Model file for the job. Use its own axes, mm. Face numbers are marked on the shaded views. A direction names the side the tool comes from. Round coordinates to 2 decimals unless told otherwise and drop trailing zeros. Loops run counter-clockwise (first coordinate to the right, second up) from the corner with the lowest first, then second, coordinate; pieces in that order, holes last. Notation, with made-up numbers: M 2.25,-29.75 L 54.25,-29.75 A19 ccw 54.25,2.25 Z; hole C -21,-37.75 d10. An arc over 180 degrees is marked long. Use a Markdown table: item, result. Add a question column.
Item 1: Saw through at B-B on x = 18.5. Write the cut outline in (y, z), then the cut area to 3 significant figures.
Item 2: Saw through at D-D on z = 48. Write the cut outline in (x, y) (3 decimals), then the cut area to 3 significant figures.
Item 3: Two-plate mould, pull along Z, no slides. Class the marked faces 1 and 2: +Z half, -Z half, draft (parallel to the pull), parting line (faces both ways), or undercut.
Item 4: Pin check, flat tips, straight feed: P1, Ø8, axis at x = 11.5, z = 59.5, coming from the -Y side; P2, Ø4, axis at y = 38.1, z = 6.35, coming from the +X side; P3, Ø10, axis at x = 17.5, z = 0.5, coming from the -Y side; P4, Ø8.5, axis at y = 38.1, z = 57.15, coming from the +X side (3 decimals). Stop position of each tip, or through.
Item 5: Saw through at C-C on z = 5. Write the cut outline in (x, y) (1 decimal), then the cut area to 3 significant figures.
Item 6: Wall check: L1, parallel to Z at x = 2.2, y = 38.1 (3 decimals); L2, parallel to Y at x = 1.2, z = 57.15 (3 decimals); L3, parallel to X at y = 22.5, z = 49 (3 decimals). Give the ranges that are in metal, low to high. Write a range as from..to.
Item 7: Saw through at A-A on y = 38.1. Write the cut outline in (x, z) (3 decimals).
Item 8: Tool access for the marked faces 3, 4 and 5: list every direction of +Z, -Z, +X, -X, +Y, -Y with a clear straight run to the whole face (end or side of a thin tool).
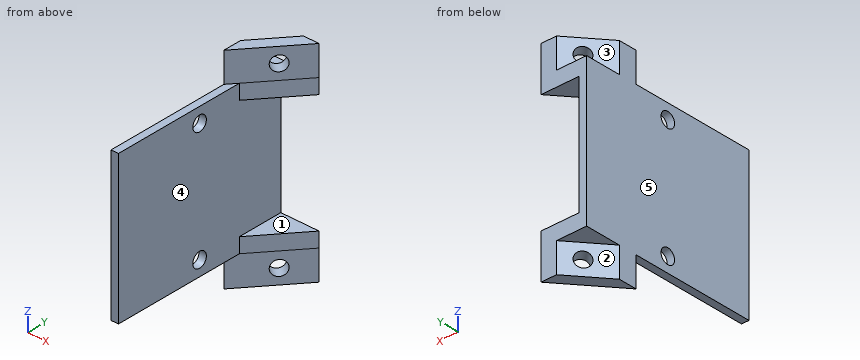
Autodesk Inventor part; units mm, degrees
ref_plane "YZ Plane" through (0, 0, 0) normal (1, 0, 0) x (0, 1, 0)
ref_plane "XZ Plane" through (0, 0, 0) normal (0, 1, 0) x (-1, 0, 0)
ref_plane "XY Plane" through (0, 0, 0) normal (0, 0, 1) x (1, 0, 0)
sketch "Sketch1" plane through (0, 0, 0) normal (1, 0, 0) x (0, 1, 0)
  line L0 (76.2, 63.5) -> (0, 63.5)
  line L1 (0, 63.5) -> (0, 0)
  line L2 (0, 0) -> (76.2, 0)
  line L3 (76.2, 0) -> (76.2, 63.5)
  dimension "d0" = 76.2
  dimension "d1" = 63.5
extrude "Extrusion1" add sketch "Sketch1" along normal blind 3.175
sketch "Sketch2" plane through (3.175, 0, 0) normal (1, 0, 0) x (0, 0, -1)
  line L0 (-63.5, 76.2) -> (-63.5, 0)
  line L1 (0, 0) -> (0, 76.2)
  line L2 (0, 76.2) -> (-63.5, 76.2)
  point P0 (-57.15, 38.1)
  point P1 (-6.35, 38.1)
  dimension "d11" = 6.35
  dimension "d12" = 6.35
  dimension "d13" = 38.1
  dimension "d14" = 38.1
hole "Hole1" at (3.175, 38.1, 57.15) at (3.175, 38.1, 6.35) direction (-1, 0, 0) diameter 6.35 end through all
sketch "Sketch3" plane through (0, 0, 0) normal (0, 0, -1) x (-1, 0, 0)
  line L0 (-19.5018, 76.2) -> (-3.175, 56.7425)
  line L1 (-3.175, 56.7425) -> (-3.175, 76.2)
  line L2 (-3.175, 0) -> (-3.175, 76.2)
  line L3 (-3.175, 76.2) -> (-19.5018, 76.2)
  line L4 (0, 76.2) -> (-3.175, 76.2)
  point P0 (0, 0)
  dimension "d15" = 40
  dimension "d18" = 25.4
extrude "Extrusion2" add sketch "Sketch3" against normal blind 6.35
sketch "Sketch4" plane through (0, 0, 0) normal (0, 0, -1) x (-1, 0, 0)
  line L0 (0, 76.2) -> (-19.5018, 76.2)
  line L1 (-19.5018, 76.2) -> (0, 52.9587)
  line L2 (-19.5018, 76.2) -> (-12.8703, 76.2)
  line L3 (-12.8703, 76.2) -> (0, 60.8617)
  line L4 (-3.175, 56.7425) -> (-19.5018, 76.2)
  line L5 (0, 52.9587) -> (0, 60.8617)
  line L6 (0, 0) -> (0, 76.2)
  point P0 (-3.175, 76.2)
  dimension "d21" = 5.08
extrude "Extrusion3" add sketch "Sketch4" along normal blind 12.7 contours L3 L5 L1 L0
ref_plane "Work Plane1" through (0, 0, 31.75) normal (0, 0, -1) x (-1, 0, 0)
mirror "Mirror1" about plane through (0, 0, 31.75) normal (0, 0, -1) of "Extrusion2", "Extrusion3"
sketch "Sketch5" plane through (12.8703, 76.2, -12.7) normal (-0.766, 0.6428, 0) x (0, 0, 1)
  line L0 (88.9, -20.0227) -> (88.9, 0)
  line L1 (76.2, -21.1374) -> (88.9, -21.1374)
  point P0 (12.7, -66.6455)
  point P1 (6.35, -8.4374)
  point P2 (82.55, -8.4374)
  point P3 (88.9, -15.0833)
  point P4 (88.9, -26.0768)
  dimension "d31" = 76.2
  dimension "d32" = 6.35
  dimension "d33" = 12.7
hole "Hole2" at (7.4469, 69.7366, -6.35) at (7.4469, 69.7366, 69.85) direction (0.766, -0.6428, 0) diameter 6.35 end through all
properties part number "conecter bracet cover plate"
Entries:
| question | item | result |
|---|---|---|
| 1 | outline | M 75.01,-12.7 L 76.2,-12.7 L 76.2,6.35 L 75.01,6.35 Z; M 75.01,57.15 L 76.2,57.15 L 76.2,76.2 L 75.01,76.2 Z |
| 1 | area | 45.5 mm2 |
| 2 | outline | M 0,0 L 3.175,0 L 3.175,76.2 L 0,76.2 Z |
| 2 | area | 242 mm2 |
| 3 | face 1 | undercut |
| 3 | face 2 | draft |
| 4 | P1 | y = 61.9 |
| 4 | P2 | through |
| 4 | P3 | y = 67.86 |
| 4 | P4 | x = 3.175 |
| 5 | outline | M 0,0 L 3.2,0 L 3.2,35.2 L 0,35.2 Z; M 0,41 L 3.2,41 L 3.2,56.7 L 19.5,76.2 L 0,76.2 Z |
| 5 | area | 383 mm2 |
| 6 | L1 | 0..3.175, 9.525..53.975, 60.325..63.5 |
| 6 | L2 | 0..34.925, 41.275..76.2 |
| 6 | L3 | 0..3.175 |
| 7 | outline | M 0,0 L 3.175,0 L 3.175,3.175 L 0,3.175 Z; M 0,9.525 L 3.175,9.525 L 3.175,53.975 L 0,53.975 Z; M 0,60.325 L 3.175,60.325 L 3.175,63.5 L 0,63.5 Z |
| 8 | face 3 | +Z, -X, +Y |
| 8 | face 4 | +X, -Y |
| 8 | face 5 | +Z, -Z, -X, +Y, -Y |
